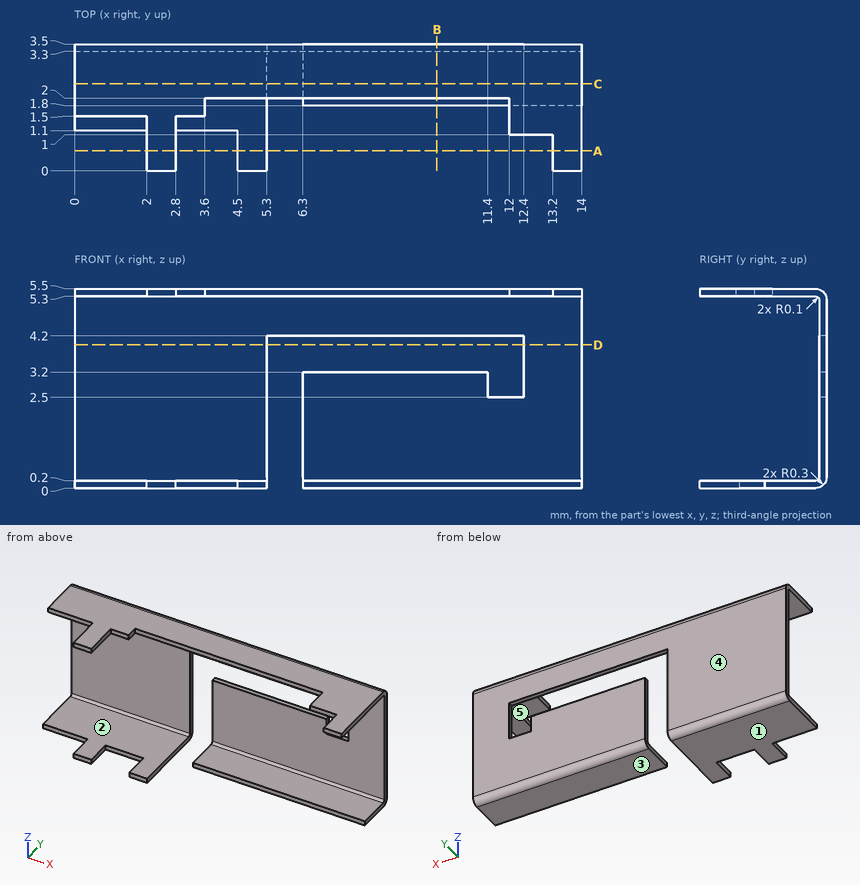
Geometry check sheet. Reference: drawing and pictorial views, mm from the part's lowest x, y, z. A direction names the side the tool comes from. Give positions to 0.01 mm unless a question says otherwise; leave off trailing zeros. Loops run counter-clockwise (first coordinate to the right, second up) from the corner with the lowest first, then second, coordinate; pieces in that order, holes last. Notation, with made-up numbers: (-22.75, 55) - (-8.75, 55) arc R22 cw to (-8.75, 82) - close; hole circle Ø5 at (-9.5, -36). An arc over 180 degrees is marked (long way). Use CSV: the item, a comma, the result in double quotes. Start each with the question number.
Q1. Scan lines: probe 1 along Z at (x, y) = (9.25, 2.05); probe 2 along Y at (x, z) = (3, 3.5); probe 3 along Z at (x, y) = (8, 1.85). Record each from-to range of solid material in increasing order. Write a range as from..to.
Q2. Access from +Z, -Z, +X, -X, +Y, -Y to the whole of each face (thin tool, end or side, straight path). Record for the marked faces 1 and 2.
Q3. Release check for a two-part mould opening along Z. For the marked faces 3, 4 and 5 record: +Z half, -Z half, draft (parallel to the pull), parting line (faces both ways), or undercut.
Q4. Section check C-C, the plane y = 2.4. Record the cut outline in (x, z).
Q5. Section check B-B, the plane x = 10. Record the cut outline in (y, z), and give its area (3 significant figures).
Q6. Section check A-A, the plane y = 0.55. Record the cut outline in (x, z).
Q7. Section check D-D, the plane z = 3.95. Record the cut outline in (x, y).
Findings below:
1,probe 1,"z = 0..0.2, 5.3..5.5"
1,probe 2,"y = 3.3..3.5"
1,probe 3,"z = 0..0.2"
2,face 1,"-Z, +X, -X, +Y, -Y"
2,face 2,"+X, -X, -Y"
3,face 3,"-Z half"
3,face 4,"draft"
3,face 5,"undercut"
4,outline,"(0, 0) - (5.3, 0) - (5.3, 0.2) - (0, 0.2) - close; (0, 5.3) - (14, 5.3) - (14, 5.5) - (0, 5.5) - close; (6.3, 0) - (14, 0) - (14, 0.2) - (6.3, 0.2) - close"
5,outline,"(1.8, 0) - (3.2, 0) arc R0.3 ccw to (3.5, 0.3) - (3.5, 3.2) - (3.3, 3.2) - (3.3, 0.3) arc R0.1 cw to (3.2, 0.2) - (1.8, 0.2) - close; (2, 5.3) - (3.2, 5.3) arc R0.1 cw to (3.3, 5.2) - (3.3, 4.2) - (3.5, 4.2) - (3.5, 5.2) arc R0.3 ccw to (3.2, 5.5) - (2, 5.5) - close"
5,area,"1.43 mm^2"
6,outline,"(2, 0) - (2.8, 0) - (2.8, 0.2) - (2, 0.2) - close; (2, 5.3) - (2.8, 5.3) - (2.8, 5.5) - (2, 5.5) - close; (4.5, 0) - (5.3, 0) - (5.3, 0.2) - (4.5, 0.2) - close; (13.2, 5.3) - (14, 5.3) - (14, 5.5) - (13.2, 5.5) - close"
7,outline,"(0, 3.3) - (5.3, 3.3) - (5.3, 3.5) - (0, 3.5) - close; (12.4, 3.3) - (14, 3.3) - (14, 3.5) - (12.4, 3.5) - close"
